For this review, use the dimensioned drawing (mm, ordinates from the lowest corner) and the shaded views. Coordinates: 2 decimals unless noted, no trailing zeros. Loops run counter-clockwise (first coordinate to the right, second up) from the corner with the lowest first, then second, coordinate; pieces in that order, holes last. Notation, with made-up numbers: (-25, -12.5) - (0, -12.5) arc R14 cw to (0, 0.5) - close; hole circle Ø10 at (79, -26). An arc over 180 degrees is marked (long way). One line per item, written item: value. Start each with the question number.
1. To check wall thickness, follow line 1 (Z direction, x = 19.05, y = 10); line 2 (Z direction, x = 19.05, y = 4); line 3 (Y direction, x = 18.5, z = 8.5). State the ranges of each line that lie inside material, in increasing order.
2. Insertion check: P1, Ø6, axis at x = 6.5, z = 27.5, coming from the -Y side; P2, Ø10, axis at x = 17.5, z = 20, coming from the -Y side; P3, Ø6, axis at x = 14, z = 8, coming from the +Y side. Each pin has a flat end and moves straight along its axis. Give the tip position at first contact, or say it passes through.
3. We need section B-B, the plane x = 19.05. Give the boundary of the cut face in (y, z).
4. We need section A-A, the plane z = 19.05. Give the boundary of the cut face in (x, y), then the cut area to 3 significant figures.
5. Mouldability with a two-part tool opening along X and no side actions: class the marked faces 1, 2 and 3 as +X half, -X half, draft (parallel to the pull), parting line (faces both ways), or undercut.
6. We need section C-C, the plane y = 44. Give the boundary of the cut face in (x, z), then the cut area to 3 significant figures.
7. We need section D-D, the plane z = 11.5. Give the boundary of the cut face in (x, y), then the cut area to 3 significant figures.
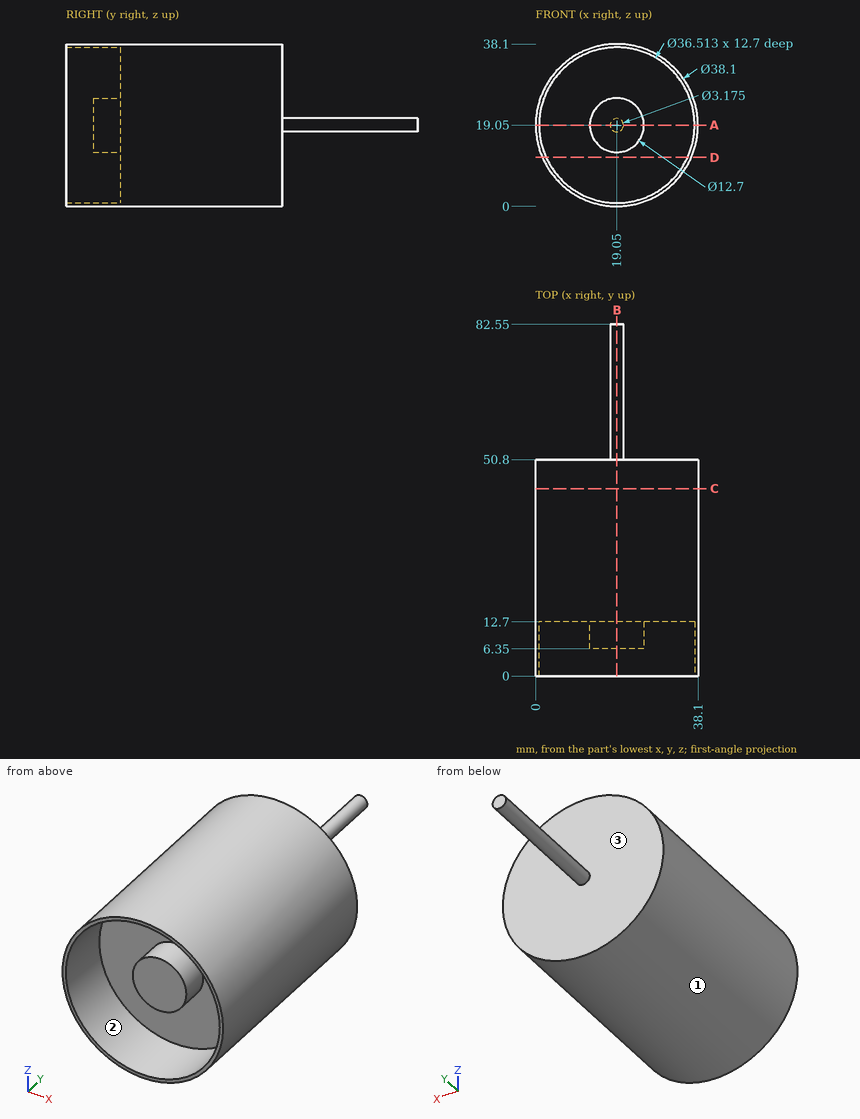
Findings below:
1. line 1: 0 to 0.79, 12.7 to 25.4, 37.31 to 38.1
1. line 2: 0 to 0.79, 37.31 to 38.1
1. line 3: 12.7 to 50.8
2. P1: y = 12.7
2. P2: y = 6.35
2. P3: y = 50.8
3. outline: (0, 0) - (50.8, 0) - (50.8, 17.46) - (82.55, 17.46) - (82.55, 20.64) - (50.8, 20.64) - (50.8, 38.1) - (0, 38.1) - (0, 37.31) - (12.7, 37.31) - (12.7, 25.4) - (6.35, 25.4) - (6.35, 12.7) - (12.7, 12.7) - (12.7, 0.79) - (0, 0.79) - close
4. outline: (0, 0) - (0.79, 0) - (0.79, 12.7) - (12.7, 12.7) - (12.7, 6.35) - (25.4, 6.35) - (25.4, 12.7) - (37.31, 12.7) - (37.31, 0) - (38.1, 0) - (38.1, 50.8) - (20.64, 50.8) - (20.64, 82.55) - (17.46, 82.55) - (17.46, 50.8) - (0, 50.8) - close
4. area: 1,650 mm2
5. face 1: parting line
5. face 2: undercut
5. face 3: draft
6. outline: circle Ø38.1 at (19.05, 19.05)
6. area: 1,140 mm2
7. outline: (1.56, 0) - (2.43, 0) - (2.43, 12.7) - (35.67, 12.7) - (35.67, 0) - (36.54, 0) - (36.54, 50.8) - (1.56, 50.8) - close
7. area: 1,350 mm2
